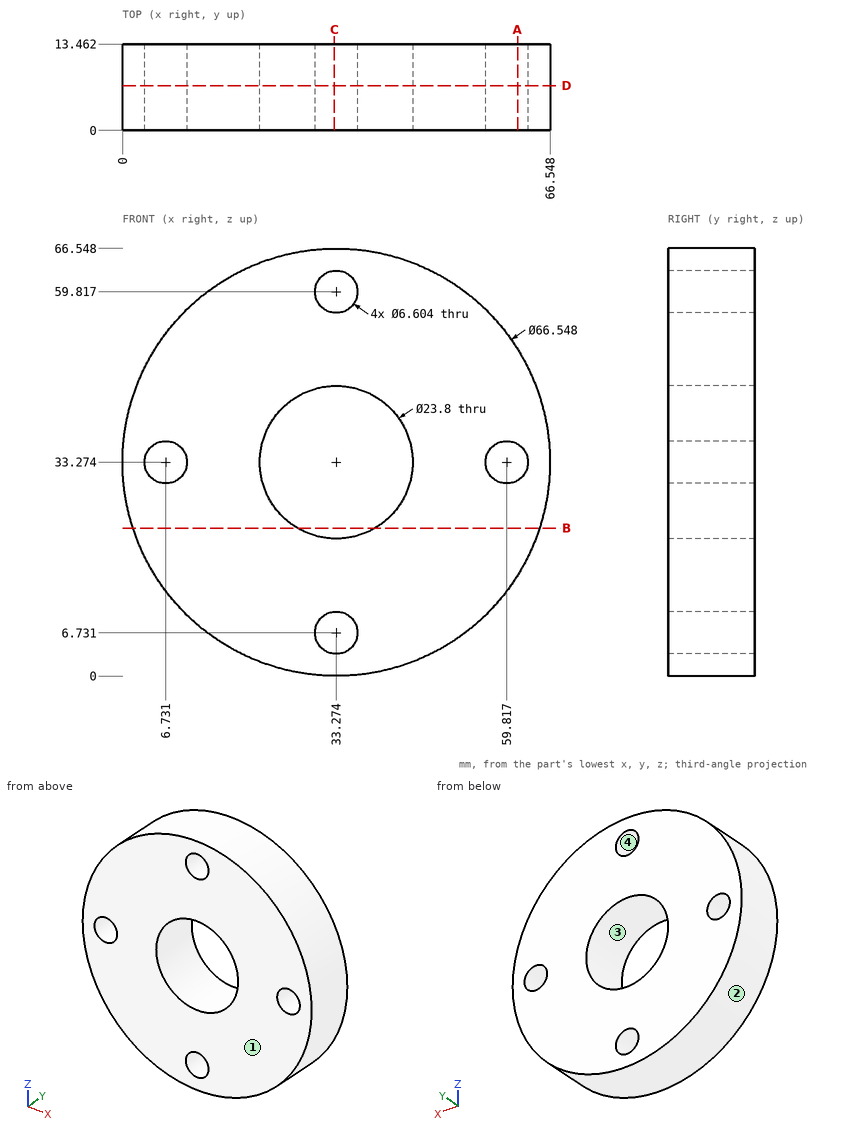
Part print with two shaded views. Sizes in mm from the minimum x, y, z corner. Round coordinates to 2 decimals unless told otherwise and drop trailing zeros. Write each loop counter-clockwise with the first axis right and the second up, starting at its lowest first coordinate (ties: lowest second). Pieces come first, ordered by that corner, then holes. Notation, with made-up numbers: M 10.5,12 L 42.5,12 A10 ccw 42.5,23 Z; hole C 16.25,-21 d5. An arc over 180 degrees is marked long. Put each result on its own line as item: value. Start each with the question number.
1) Saw through at C-C, the plane x = 33. Write the cut outline in (y, z), and give its area (3 significant figures).
2) Pull direction Z, two halves, no side cores. Call the marked faces 1, 2, 3 and 4: pulls with the +Z half, pulls with the -Z half, needs draft (parallel to the pull), parting line crosses it, or undercut.
3) Pin check, flat tips, straight feed: pin 1 Ø3 at (y, z) = (1.5, 39.5) entering from -X; pin 2 Ø4 at (x, z) = (59.817, 33.274) entering from -Y; pin 3 Ø5 at (x, y) = (30.5, 8) entering from +Z; pin 4 Ø8 at (x, y) = (40, 8.5) entering from +Z. Stop position of each tip, or through.
4) Drill centre lines: probe 1 along X at (y, z) = (6.25, 43) (1 decimal); probe 2 along X at (y, z) = (12, 29) (1 decimal); probe 3 along Z at (x, y) = (28.5, 9) (1 decimal). Where is each one in solid material? Low to high. Write a range as [from, to].
5) Saw through at B-B, the plane z = 23. Write the cut outline in (x, y).
6) Saw through at D-D, the plane y = 7. Write the cut outline in (x, z) (1 decimal), and give its area (3 significant figures).
7) Saw through at A-A, the plane x = 61.5. Write the cut outline in (y, z) (1 decimal).
Resolved:
1. outline: M 0,0 L 13.46,0 L 13.46,3.44 L 0,3.44 Z; M 0,10.02 L 13.46,10.02 L 13.46,21.38 L 0,21.38 Z; M 0,45.17 L 13.46,45.17 L 13.46,56.53 L 0,56.53 Z; M 0,63.11 L 13.46,63.11 L 13.46,66.55 L 0,66.55 Z
1. area: 398 mm²
2. face 1: needs draft
2. face 2: parting line crosses it
2. face 3: undercut
2. face 4: undercut
3. pin 1: x = 0.34
3. pin 2: through
3. pin 3: z = 66.55
3. pin 4: z = 66.44
4. probe 1: [1.5, 26.4], [40.1, 65.1]
4. probe 2: [0.3, 22.2], [44.4, 66.3]
4. probe 3: [0.3, 22.4], [44.2, 66.2]
5. outline: M 1.63,0 L 27.27,0 L 27.27,13.46 L 1.63,13.46 Z; M 39.28,0 L 64.92,0 L 64.92,13.46 L 39.28,13.46 Z
6. outline: C 33.3,33.3 d66.5; hole C 6.7,33.3 d6.6; hole C 33.3,33.3 d23.8; hole C 33.3,6.7 d6.6; hole C 33.3,59.8 d6.6; hole C 59.8,33.3 d6.6
6. area: 2,900 mm²
7. outline: M 0,15.7 L 13.5,15.7 L 13.5,30.4 L 0,30.4 Z; M 0,36.1 L 13.5,36.1 L 13.5,50.9 L 0,50.9 Z
